from build123d import *

# Parameters (mm, degrees)
F1_DEPTH  = 2
F2_R      = 2.5
F3_DEPTH  = 3
F4_R      = 1.4
F5_DEPTH  = 3
F6_R      = 1.4
F7_DEPTH  = 3
F8_R      = 1.4
F9_DEPTH  = 3.1
F10_R     = 1.4
F11_DEPTH = 3
F12_R     = 2.65
F12_W     = 54.34
F12_H     = 69.58
F13_DEPTH = 6.65
F14_R     = 1.75
F14_R_2   = 1.4
F15_DEPTH = 25
F16_W     = 13.04
F16_H     = 2.13
F16_W_2   = 10
F16_H_2   = 2.5
F17_DEPTH = 3
F18_SIZE  = 1


with BuildPart() as f1:
    # F0 (on Top) → F1 (new body)
    with BuildSketch(Plane.XY):
        with BuildLine():
            Line((55.84, 71.08), (-2.5, 71.08))
            ThreePointArc((-2.5, 71.08), (-8.156854, 68.736854), (-10.5, 63.08))
            Line((-10.5, 63.08), (-10.5, 5.5))
            ThreePointArc((-10.5, 5.5), (-8.156854, -0.156854), (-2.5, -2.5))
            Line((-2.5, -2.5), (55.84, -2.5))
            ThreePointArc((55.84, -2.5), (61.496854, -0.156854), (63.84, 5.5))
            Line((63.84, 5.5), (63.84, 63.08))
            ThreePointArc((63.84, 63.08), (61.496854, 68.736854), (55.84, 71.08))
        make_face()
    extrude(amount=F1_DEPTH)

    # F2 (on face) → F3 (join)
    with BuildSketch(Plane.XY.offset(2)):
        with Locations((17.78, 66.04)):
            Circle(F2_R)
        with Locations((45.72, 66.04)):
            Circle(F2_R)
        with Locations((2.54, 15.24)):
            Circle(F2_R)
        with Locations((50.8, 13.97)):
            Circle(F2_R)
    extrude(amount=F3_DEPTH)

    # F4 (on face) → F5 (join)
    with BuildSketch(Plane.XY.offset(5)):
        with Locations((17.78, 66.04)):
            Circle(F4_R)
    extrude(amount=F5_DEPTH)

    # F6 (on face) → F7 (join)
    with BuildSketch(Plane.XY.offset(5)):
        with Locations((45.72, 66.04)):
            Circle(F6_R)
    extrude(amount=F7_DEPTH)

    # F8 (on face) → F9 (join)
    with BuildSketch(Plane.XY.offset(5)):
        with Locations((2.54, 15.24)):
            Circle(F8_R)
    extrude(amount=F9_DEPTH)

    # F10 (on face) → F11 (join)
    with BuildSketch(Plane.XY.offset(5)):
        with Locations((50.8, 13.97)):
            Circle(F10_R)
    extrude(amount=F11_DEPTH)

    # F12 (on face) → F13 (join)
    with BuildSketch(Plane.XY.offset(2)):
        with BuildLine():
            ThreePointArc((-2.5, 71.08), (-8.156854, 68.736854), (-10.5, 63.08))
            Line((-10.5, 63.08), (-10.5, 5.5))
            ThreePointArc((-10.5, 5.5), (-8.156854, -0.156854), (-2.5, -2.5))
            Line((-2.5, -2.5), (55.84, -2.5))
            ThreePointArc((55.84, -2.5), (61.496854, -0.156854), (63.84, 5.5))
            Line((63.84, 5.5), (63.84, 63.08))
            ThreePointArc((63.84, 63.08), (61.496854, 68.736854), (55.84, 71.08))
            Line((55.84, 71.08), (-2.5, 71.08))
        make_face()
        with Locations((-5.5, 16.5)):
            Circle(F12_R, mode=Mode.SUBTRACT)
        with Locations((58.84, 16.5)):
            Circle(F12_R, mode=Mode.SUBTRACT)
        with Locations((-5.5, 52.08)):
            Circle(F12_R, mode=Mode.SUBTRACT)
        with Locations((26.67, 34.29)):
            Rectangle(F12_W, F12_H, mode=Mode.SUBTRACT)
        with Locations((58.84, 52.08)):
            Circle(F12_R, mode=Mode.SUBTRACT)
    extrude(amount=F13_DEPTH)

    # F14 (on face) → F15 (cut)
    with BuildSketch(Plane.XY.offset(8.65)):
        with Locations((-5.5, 9.5)):
            Circle(F14_R)
        with Locations((-4.5, 2.5)):
            Circle(F14_R_2)
        with Locations((-4.5, 66.08)):
            Circle(F14_R_2)
        with Locations((-5.5, 59.08)):
            Circle(F14_R)
        with Locations((57.84, 66.08)):
            Circle(F14_R_2)
        with Locations((58.84, 59.08)):
            Circle(F14_R)
        with Locations((58.84, 9.5)):
            Circle(F14_R)
        with Locations((57.84, 2.5)):
            Circle(F14_R_2)
    extrude(amount=-F15_DEPTH, mode=Mode.SUBTRACT)

    # F16 (on face) → F17 (cut)
    with BuildSketch(Plane.XZ.offset(2.5)):
        with Locations((15.02, 7.585)):
            Rectangle(F16_W, F16_H)
        with Locations((45.34, 7.4)):
            Rectangle(F16_W_2, F16_H_2)
    extrude(amount=-F17_DEPTH, mode=Mode.SUBTRACT)

    # F18
    f18_edges = [f1.edges().sort_by_distance(p)[0] for p in [
        (56.19, 16.5, 8.65),
        (56.19, 52.08, 8.65),
        (-8.15, 52.08, 8.65),
        (-8.15, 16.5, 8.65),
    ]]
    chamfer(f18_edges, length=F18_SIZE)


solid = f1.part
Build history of the part. All positions in model axes, mm. A direction names the side the tool comes from. Round coordinates to 2 decimals unless told otherwise and drop trailing zeros. Write each loop counter-clockwise with the first axis right and the second up, starting at its lowest first coordinate (ties: lowest second). Pieces come first, ordered by that corner, then holes. Notation, with made-up numbers: M -37,52.5 L 7,52.5 A22 ccw 7,80.5 Z; hole C 36,-30.75 d3. An arc over 180 degrees is marked long. Answer as a JSON object with one key per item and string values. Group by question number.
(1) Mould opens along X. For faces 4 (the flat face through (4, 14, 5)), 5 (the flat face through (26, -2.5, 4)), 6 (the cylindrical face through (61.559, 68.674, 4.264)) say: pulls with the +X half, pulls with the -X half, needs draft (parallel to the pull), parting line crosses it, or undercut.
(2) Cut at B-B (y = 41). Give the cut face in (x, z).
(3) Cut at A-A (x = 2.54). Give the cut face in (y, z).
(4) Which spindle directions (+Z, -Z, +X, -X, +Y, -Y) get a long thin tool onto all of the face, cutting with end or side? Do faces 1 (the cylindrical face through (-3.85, 1.26, 4.39)), 2 (the cylindrical face through (61.368, 17.296, 4.785)), 3 (the flat face through (45, -2, 6.15)). Say none if no direction does.
(5) Flat gauge pins, fed straight in: pin 1 (4 mm diameter, centred on x = 50, y = 15, fed in from +Z); pin 2 (1 mm diameter, centred on y = -1, z = 7.5, fed in from +X); pin 3 (5 mm diameter, centred on x = -5.5, y = 52.08, fed in from -Z); pin 4 (5.5 mm diameter, centred on x = 3, y = 14, fed in from +Z). Where does each tip first touch, or does it go through?
(6) Cut at C-C (x = 45.72). Give the cut face in (y, z).
(7) Drill centre lines: L1, parallel to Y at x = 19.5, z = 4; L2, parallel to Y at x = 10, z = 5.75; L3, parallel to X at y = 61.5, z = 3.25. Where is each one in solid material? Low to high.
Responses:
{
 "1": {"face 4": "undercut", "face 5": "needs draft", "face 6": "pulls with the +X half"},
 "2": {"outline": "M -10.5,0 L 63.84,0 L 63.84,8.65 L 53.84,8.65 L 53.84,2 L -0.5,2 L -0.5,8.65 L -10.5,8.65 Z"},
 "3": {"outline": "M -2.5,0 L 71.08,0 L 71.08,8.65 L 69.08,8.65 L 69.08,2 L 17.74,2 L 17.74,5 L 16.64,5 L 16.64,8.1 L 13.84,8.1 L 13.84,5 L 12.74,5 L 12.74,2 L -0.5,2 L -0.5,8.65 L -2.5,8.65 Z"},
 "4": {"face 1": "+Z, -Z", "face 2": "+Z", "face 3": "+Z, -Y"},
 "5": {"pin 1": "stops at z = 8", "pin 2": "stops at x = 61.13", "pin 3": "stops at z = 0", "pin 4": "stops at z = 8.1"},
 "6": {"outline": "M -2.5,0 L 71.08,0 L 71.08,8.65 L 69.08,8.65 L 69.08,2 L 68.54,2 L 68.54,5 L 67.44,5 L 67.44,8 L 64.64,8 L 64.64,5 L 63.54,5 L 63.54,2 L -0.5,2 L -0.5,6.15 L -2.5,6.15 Z"},
 "7": {"L1": "y = -2.5 to -0.5, 64.23 to 67.85, 69.08 to 71.08", "L2": "y = -2.5 to -0.5, 69.08 to 71.08", "L3": "x = -10.5 to -0.5, 53.84 to 63.84"}
}
